```python
from build123d import *

# Parameters (mm, degrees)
PAD_DEPTH       = 15
SKETCH002_R     = 71
POCKET_DEPTH    = 13.5
POCKET001_DEPTH = 13.5
PAD001_DEPTH    = 35
PAD002_DEPTH    = 35
SKETCH_R        = 9.6
POCKET002_DEPTH = 41.1514534441
SKETCH009_R     = 9.6
POCKET003_DEPTH = 97.4839978397


with BuildPart() as part:
    # Sketch001 → Pad (new body)
    with BuildSketch(Plane.XY):
        with BuildLine():
            ThreePointArc((71.2460525222, 20), (44.7436533058, 58.9406946756), (0.1121090023, 73.9999150781))
            Line((0.1121090023, 73.9999150781), (-70, 74.1061334774))
            ThreePointArc((-69.9999999999, 74.1061334774), (-89.3215614177, 42.9266570301), (-52.7907882568, 39.6122793491))
            ThreePointArc((63.5437766663, 17.8378375087), (12.1424161228, 64.8734285413), (-52.7907882568, 39.6122793491))
            ThreePointArc((63.5437766663, 17.8378375087), (68.4759958054, 15.0677809492), (71.2460525222, 20))
        make_face()
    extrude(amount=PAD_DEPTH)

    # Sketch002 → Pocket (cut)
    with BuildSketch(Plane(origin=(0, 0, 0), x_dir=(1, 0, 0), z_dir=(0, 0, -1))):
        Circle(SKETCH002_R)
    extrude(amount=-POCKET_DEPTH, mode=Mode.SUBTRACT)

    # Sketch003 → Pocket001 (cut)
    with BuildSketch(Plane(origin=(0, 0, 0), x_dir=(1, 0, 0), z_dir=(0, 0, -1))):
        Polygon((-153.2491449427, -71.2322507725), (0.107679068, -70.9999183467), (-35.4631, 35.7409), align=None)
    extrude(amount=-POCKET001_DEPTH, mode=Mode.SUBTRACT)

    # Sketch005 → Pad001 (new body)
    with BuildSketch(Plane.XY.offset(15)):
        Polygon((38.5306472975, 61.493001381), (45.4772310021, 68.6863993843), (67.0574250122, 47.8466482706), (60.1108413076, 40.6532502672), align=None)
    extrude(amount=-PAD001_DEPTH)

    # Sketch006 → Pad002 (new body)
    with BuildSketch(Plane.XY.offset(15)):
        Polygon((-41.8276469497, 71.0634495008), (-43.8797678097, 76.7016052255), (-15.6889891861, 86.9622095253), (-9.8847001983, 71.0150565952), align=None)
    extrude(amount=-PAD002_DEPTH)

    # Sketch → Pocket002 (cut, through all)
    with BuildSketch(Plane(origin=(49.3207443026, 51.0731258241, 0), x_dir=(0.7193398003, -0.6946583705, 0), z_dir=(-0.6946583705, -0.7193398003, 0))):
        with Locations((0, -20)):
            Circle(SKETCH_R)
    extrude(amount=-POCKET002_DEPTH, mode=Mode.SUBTRACT)

    # Sketch009 → Pocket003 (cut, through all)
    with BuildSketch(Plane(origin=(-29.7843784979, 81.8319073754, 0), x_dir=(-0.9396926208, -0.3420201433, 0), z_dir=(-0.3420201433, 0.9396926208, 0))):
        with Locations((0, -20)):
            Circle(SKETCH009_R)
    extrude(amount=-POCKET003_DEPTH, mode=Mode.SUBTRACT)


solid = part.part
```
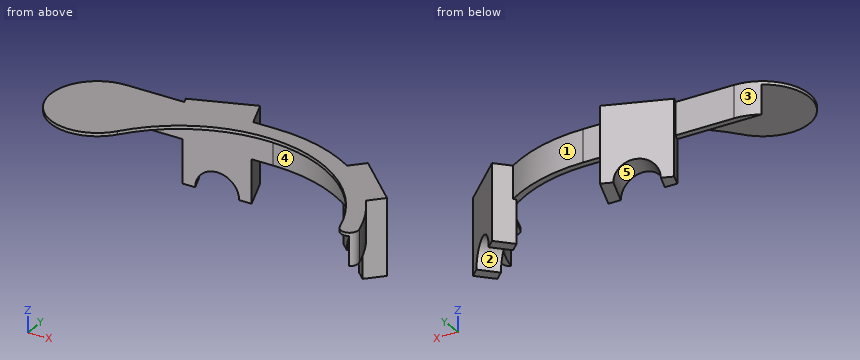
Input: part model. Units: mm. Frame: model coordinates. Face numbers are marked on the shaded views. A direction names the side the tool comes from. Give positions to 0.01 mm unless a question says otherwise; leave off trailing zeros. Order: outer loops, then holes, each group sorted by start corner. A loop starts at its lowest first (then second) coordinate and runs counter-clockwise, first axis right, second up. Notation, with made-up numbers: (53.25, 67) - (87.25, 67) arc R18 ccw to (87.25, 93) - close; hole circle Ø8 at (5.25, 68). An arc over 180 degrees is marked (long way). One line per item, written item: value.
1. Pin query (flat end, axial travel): pin 1 Ø17.5 at (x, y) = (56.5, 28.5) entering from -Z; pin 2 Ø1.5 at (x, z) = (-59.5, 8) entering from +Y; pin 3 Ø4 at (x, z) = (-28, -1.5) entering from -Y. Return the tip coordinate at first contact, or that it passes through.
Determined:
pin 1: z = 0
pin 2: y = 74.09
pin 3: y = 71.04
2. Cut plane B-B, the plane z = -16. Output: boundary loops of the cut face in (x, y), and give its area (3 significant figures).
Determined:
outline: (-43.88, 76.7) - (-41.83, 71.06) - (-35.15, 71.05) - (-37.99, 78.85) - close; (-21.58, 84.82) - (-16.56, 71.03) - (-9.88, 71.02) - (-15.69, 86.96) - close; (38.53, 61.49) - (43.04, 57.14) - (49.99, 64.33) - (45.48, 68.69) - close; (55.6, 45.01) - (60.11, 40.65) - (67.06, 47.85) - (62.54, 52.2) - close
area: 270 mm2
3. Cut plane A-A, the plane z = -2. Output: boundary loops of the cut face in (x, y), and give its area (3 significant figures).
Determined:
outline: (-43.88, 76.7) - (-41.83, 71.06) - (-9.88, 71.02) - (-15.69, 86.96) - close; (38.53, 61.49) - (60.11, 40.65) - (67.06, 47.85) - (45.48, 68.69) - close
area: 645 mm2
4. Cut plane D-D, the plane x = -57. Output: boundary loops of the cut face in (y, z).
Determined:
outline: (35.38, 13.5) - (71.09, 13.5) - (71.09, 0) - (74.09, 0) - (74.09, 15) - (35.38, 15) - close
5. Reachability of the marked faces 4 and 5 from +Z, -Z, +X, -X, +Y, -Y: full face, straight path, thin tool, end or side. Return the list, or none.
Determined:
face 4: -Z, -X, -Y
face 5: -Z
6. Draft query along Y for the marked faces 1, 2 and 3. Return one class per face: released by +Y, released by -Y, zero draft, split by the parting line, or undercut.
Determined:
face 1: released by +Y
face 2: undercut
face 3: split by the parting line
7. Line query: probe 1 along Z at (x, y) = (-49, 53); probe 2 along Y at (x, z) = (-10, 2); probe 3 along Z at (x, y) = (37, 64). Output: solid intervals per line, ascending.
Determined:
probe 1: 13.5 to 15
probe 2: 71.02 to 74.02
probe 3: 0 to 15
8. Cut plane C-C, the plane x = 13. Output: boundary loops of the cut face in (y, z), and give its area (3 significant figures).
Determined:
outline: (64.71, 13.5) - (69.8, 13.5) - (69.8, 0) - (72.85, 0) - (72.85, 15) - (64.71, 15) - close
area: 53.4 mm2
